For this review, take the finished solid that the model builds, in its own axes (mm). Give positions to 0.01 mm unless a question says otherwise; leave off trailing zeros. Write each loop counter-clockwise with the first axis right and the second up, starting at its lowest first coordinate (ties: lowest second). Pieces come first, ordered by that corner, then holes.
from build123d import *

# Parameters (mm, degrees)
SKETCH_1_R          = 2.65
EXTRUDE_1_DEPTH     = 102
SKETCH_3_R          = 43
CUT_EXTRUDE_1_DEPTH = 123.184287042


with BuildPart() as part:
    # 草图1 → 凸台-拉伸1 (new body)
    with BuildSketch(Plane(origin=(0, 0, 0), x_dir=(1, 0, 0), z_dir=(0, 1, 0))):
        with BuildLine():
            Line((-40, 45), (40, 45))
            ThreePointArc((40, 45), (47.071067812, 42.071067812), (50, 35))
            Line((50, 35), (50, -35))
            ThreePointArc((50, -35), (47.071067812, -42.071067812), (40, -45))
            Line((40, -45), (-40, -45))
            ThreePointArc((-40, -45), (-47.071067812, -42.071067812), (-50, -35))
            Line((-50, -35), (-50, 35))
            ThreePointArc((-50, 35), (-47.071067812, 42.071067812), (-40, 45))
        make_face()
        with Locations(Location((-40, 35, 0), (0, 0, 270))):
            Circle(SKETCH_1_R, mode=Mode.SUBTRACT)
        with Locations(Location((40, 35, 0), (0, 0, 90))):
            Circle(SKETCH_1_R, mode=Mode.SUBTRACT)
        with Locations(Location((40, -35, 0), (0, 0, 270))):
            Circle(SKETCH_1_R, mode=Mode.SUBTRACT)
        with Locations(Location((-40, -35, 0), (0, 0, 90))):
            Circle(SKETCH_1_R, mode=Mode.SUBTRACT)
    extrude(amount=EXTRUDE_1_DEPTH)

    # 草图3 → 切除-拉伸1 (cut, through all)
    with BuildSketch(Plane(origin=(0, 102, 0), x_dir=(1, 0, 0), z_dir=(0, 1, 0))):
        with Locations(Location((0, 0, 0), (0, 0, 270))):
            Circle(SKETCH_3_R)
    extrude(amount=-CUT_EXTRUDE_1_DEPTH, mode=Mode.SUBTRACT)


solid = part.part
(1) For L1, parallel to X at y = 46, z = 35; L2, parallel to Z at x = -39, y = 72.5; L3, parallel to X at y = 95, z = -27.5, list the stretches that pass through material, from the lowest coordinate up.
(2) We need section B-B (z = 0). Write out the cut boundary in (x, y), and give its area (3 significant figures).
(3) We need section C-C (y = 33). Write out the cut boundary in (x, z), and give its area (3 significant figures).
(4) We need section A-A (x = 35). Write out the cut boundary in (y, z).
(5) The part is to be moulded in two halves that separate along X. For faces 1 (the flat face through (-50, 50, 0)), 2 (the cylindrical face through (-41.791, 50.286, 36.953)), 3 (the flat face through (1, 50, 45)), 4 (the cylindrical face through (-38.209, 50.286, -36.953)), say which applies: +X half, -X half, draft (parallel to the pull), parting line (faces both ways), or undercut.
The answers:
1. L1: x = -50 to -42.65, -37.35 to -24.98, 24.98 to 37.35, 42.65 to 50
1. L2: z = -45 to -37.45, -32.55 to -18.11, 18.11 to 32.55, 37.45 to 45
1. L3: x = -50 to -33.06, 33.06 to 50
2. outline: (-50, 0) - (-43, 0) - (-43, 102) - (-50, 102) - close; (43, 0) - (50, 0) - (50, 102) - (43, 102) - close
2. area: 1,430 mm2
3. outline: (-50, -35) arc R10 ccw to (-40, -45) - (40, -45) arc R10 ccw to (50, -35) - (50, 35) arc R10 ccw to (40, 45) - (-40, 45) arc R10 ccw to (-50, 35) - close; hole circle Ø86 at (0, 0); hole circle Ø5.3 at (-40, -35); hole circle Ø5.3 at (-40, 35); hole circle Ø5.3 at (40, -35); hole circle Ø5.3 at (40, 35)
3. area: 3,020 mm2
4. outline: (0, -45) - (102, -45) - (102, -24.98) - (0, -24.98) - close; (0, 24.98) - (102, 24.98) - (102, 45) - (0, 45) - close
5. face 1: -X half
5. face 2: undercut
5. face 3: draft
5. face 4: undercut
